Build history of the part. All positions in model axes, mm. Give positions to 0.01 mm unless a question says otherwise; leave off trailing zeros. Write each loop counter-clockwise with the first axis right and the second up, starting at its lowest first coordinate (ties: lowest second). Pieces come first, ordered by that corner, then holes. Notation, with made-up numbers: (28.5, 79.5) -> (79.5, 79.5) arc R23 cw to (79.5, 114.5) -> close; hole circle Ø2 at (20, 27.25). An arc over 180 degrees is marked (long way). One line per question, with ' | ' between items. Start each with the question number.
(1) Band-saw the part on B-B, the plane y = 3.3. Count the separate pieces of the cut face and the enclosed holes in it, and give its area (3 significant figures).
(2) Pin check, flat tip, straight feed: P1, Ø5, axis at x = -54, z = -63.5, coming from the +Y side. Stop position of the tip, or through.
(3) Drill centre lines: probe 1 along Z at (x, y) = (-54, 3.8); probe 2 along X at (y, z) = (2.4, -41.5); probe 3 along X at (y, z) = (1.8, -38.5). Where is each one in solid material? Low to high. Write a range as from..to.
(4) Band-saw the part on C-C, the plane x = 54. Give the cut face in (y, z), and give its area (4 significant figures).
(5) Band-saw the part on A-A, the plane x = -20. Give the cut face in (y, z).
Autodesk Fusion 360 part; units mm, degrees
sketch "Plate" plane through (0, 0, 0) normal (0, 1, 0) x (1, 0, 0)
  line L0 (-54, 41.5) -> (54, 41.5) construction
  circle A0 centre (-54, 41.5) radius 3.25
  circle A1 centre (-20, 62.5) radius 2.1
  circle A2 centre (-54, 63.5) radius 3.25
  circle A3 centre (-20, 38.5) radius 2.1
  line L1 (20, 62.5) -> (-20, 62.5) construction
  line L2 (-20, 38.5) -> (20, 38.5) construction
  line L3 (-20, 62.5) -> (-20, 38.5) construction
  line L4 (54, 41.5) -> (54, 63.5) construction
  line L5 (20, 38.5) -> (20, 62.5) construction
  line L6 (54, 63.5) -> (-54, 63.5) construction
  circle A4 centre (54, 63.5) radius 3.25
  circle A5 centre (20, 38.5) radius 2.1
  circle A6 centre (20, 62.5) radius 2.1
  circle A7 centre (54, 41.5) radius 3.25
  line L7 (-54, 63.5) -> (-54, 41.5) construction
  line L8 (-62, 22.5) -> (62, 22.5)
  line L9 (62, 22.5) -> (62, 72.5)
  line L10 (62, 72.5) -> (-62, 72.5)
  line L11 (-62, 72.5) -> (-62, 22.5)
  point P0 (-54.1427, 52.5)
  dimension "d1" = 108
  dimension "d2" = 22
  dimension "d3" = 6.5
  dimension "d4" = 6.5
  dimension "d5" = 6.5
  dimension "d6" = 6.5
  dimension "d7" = 40
  dimension "d8" = 24
  dimension "d9" = 3
  dimension "d10" = 4.2
  dimension "d11" = 4.2
  dimension "d12" = 4.2
  dimension "d13" = 4.2
  dimension "d14" = 124
  dimension "d15" = 50
  dimension "d16" = 8
  dimension "d17" = 7.5
  dimension "d18" = 10
extrude "Extrude1" add sketch "Plate" along normal blind 6 makes body 1
copy_body "Body->Comp1" bodies 1 removing the originals makes body 2 in component "Plate"
chamfer "Chamfer1" distance 0.5 angle 45 28 edges at (-62, 0, -47.5) (-62, 3, -22.5) (0, 0, -22.5) (0, 6, -22.5) (62, 3, -22.5) (62, 0, -47.5) (62, 6, -47.5) (0, 0, -72.5) (62, 3, -72.5) (0, 6, -72.5) (-62, 6, -47.5) (-62, 3, -72.5) (-57.0301, 6, -64.6753) (-57.0301, 6, -42.6753) (-21.9579, 6, -39.2594) (-21.9579, 6, -63.2594) (18.0421, 6, -39.2594) (18.0421, 6, -63.2594) (50.9699, 6, -42.6753) (50.9699, 6, -64.6753) (-57.0301, 0, -64.6753) (-57.0301, 0, -42.6753) (-21.9579, 0, -39.2594) (-21.9579, 0, -63.2594) (18.0421, 0, -39.2594) (18.0421, 0, -63.2594) (50.9699, 0, -42.6753) (50.9699, 0, -64.6753) on bodies 2 in component "Plate"
component "Plate" placed x (1, 0, 0) y (0, 1, 0) z (0, 0, 1) at (0, 0, 0)
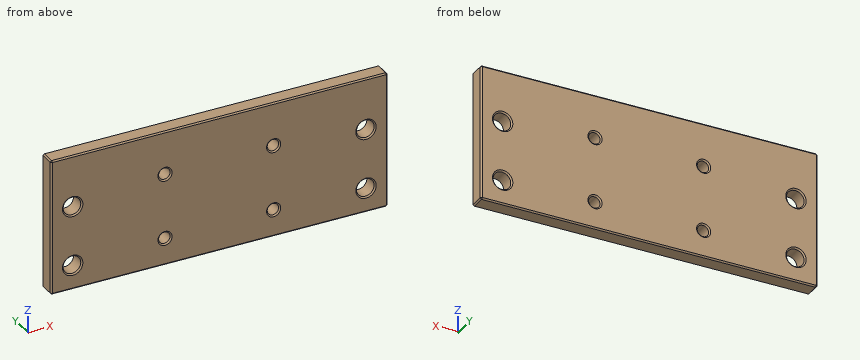
Results:
1) separate pieces: 1 | enclosed holes: 8 | area: 6,010 mm²
2) P1: passes through
3) probe 1: z = -72.5..-66.75, -60.25..-44.75, -38.25..-22.5 | probe 2: x = -62..-57.25, -50.75..50.75, 57.25..62 | probe 3: x = -62..-55.25, -52.75..-22.1, -17.9..17.9, 22.1..52.75, 55.25..62
4) outline: (0, -72) -> (0.5, -72.5) -> (5.5, -72.5) -> (6, -72) -> (6, -67.25) -> (5.5, -66.75) -> (0.5, -66.75) -> (0, -67.25) -> close; (0, -59.75) -> (0.5, -60.25) -> (5.5, -60.25) -> (6, -59.75) -> (6, -45.25) -> (5.5, -44.75) -> (0.5, -44.75) -> (0, -45.25) -> close; (0, -37.75) -> (0.5, -38.25) -> (5.5, -38.25) -> (6, -37.75) -> (6, -23) -> (5.5, -22.5) -> (0.5, -22.5) -> (0, -23) -> close | area: 220.5 mm²
5) outline: (0, -72) -> (0.5, -72.5) -> (5.5, -72.5) -> (6, -72) -> (6, -65.1) -> (5.5, -64.6) -> (0.5, -64.6) -> (0, -65.1) -> close; (0, -59.9) -> (0.5, -60.4) -> (5.5, -60.4) -> (6, -59.9) -> (6, -41.1) -> (5.5, -40.6) -> (0.5, -40.6) -> (0, -41.1) -> close; (0, -35.9) -> (0.5, -36.4) -> (5.5, -36.4) -> (6, -35.9) -> (6, -23) -> (5.5, -22.5) -> (0.5, -22.5) -> (0, -23) -> close
